```python
from build123d import *

# Parameters (mm, degrees)
SKETCH4_R                = 4.7625
SKETCH4_R_2              = 3.5179
BOSS_EXTRUDE1_DEPTH      = 12.7
BEND_1_OUTLINE_R         = 4.7625
BEND_1_OUTLINE_R_2       = 3.5179
BEND_1_ANGLE             = 90
SKETCH6_R                = 4.7625
SKETCH6_R_2              = 3.5179
POST_BEND_1_LENGTH_DEPTH = 25.4


# Read off the part's stored shape, not the designer's step: Bend 1
with BuildPart() as part:
    # Sketch4 → Boss-Extrude1 (new, symmetric)
    with BuildSketch(Plane(origin=(0, 0, 0), x_dir=(0, 0, -1), z_dir=(1, 0, 0))):
        Circle(SKETCH4_R)
        Circle(SKETCH4_R_2, mode=Mode.SUBTRACT)
    extrude(amount=BOSS_EXTRUDE1_DEPTH, both=True)

    # Bend 1 outline → Bend 1 (revolve)
    with BuildSketch(Plane(origin=(12.7, 0, 11.1125), x_dir=(1, 0, 0), z_dir=(0, 0, 1))):
        with Locations((11.1125, 0)):
            Circle(BEND_1_OUTLINE_R)
        with Locations((11.1125, 0)):
            Circle(BEND_1_OUTLINE_R_2, mode=Mode.SUBTRACT)
    revolve(axis=Axis((12.7, 0, 11.1125), (0, 1, 0)), revolution_arc=BEND_1_ANGLE)

    # Sketch6 → Post Bend 1 Length (add)
    with BuildSketch(Plane.XY.offset(11.1125)):
        with Locations((23.8125, 0)):
            Circle(SKETCH6_R)
        with Locations((23.8125, 0)):
            Circle(SKETCH6_R_2, mode=Mode.SUBTRACT)
    extrude(amount=POST_BEND_1_LENGTH_DEPTH)


solid = part.part
```
Source: CAD feature listing. Evaluate the final solid. Frame: model axes, mm. A direction names the side the tool comes from. Round coordinates to 2 decimals unless told otherwise and drop trailing zeros. Loops run counter-clockwise (first coordinate to the right, second up) from the corner with the lowest first, then second, coordinate; pieces in that order, holes last. Notation, with made-up numbers: (-27.5, 38) - (-11.5, 38) arc R38 cw to (-11.5, 76) - close; hole circle Ø9 at (76.25, 72). An arc over 180 degrees is marked (long way). Use CSV: the item, a comma, the result in double quotes.
Q1. Section query B-B, the plane z = 19.5. Output: boundary loops of the cut face in (x, y) (1 decimal), then the cut area to 3 significant figures.
Reported:
outline,"circle Ø9.5 at (23.8, 0); hole circle Ø7 at (23.8, 0)"
area,"32.4 mm^2"
Q2. Ray query, line 1 along Z through (x, y) = (-6, -0.25); line 2 along Y through (x, z) = (-3, 0); line 3 along X through (y, z) = (-0.25, 25.5). Return the intervals inside material, ascending.
Reported:
line 1,"-4.76 to -3.51, 3.51 to 4.76"
line 2,"-4.76 to -3.52, 3.52 to 4.76"
line 3,"19.06 to 20.3, 27.32 to 28.57"
Q3. Section query C-C, the plane y = 3. Output: boundary loops of the cut face in (x, z).
Reported:
outline,"(-12.7, -3.7) - (12.7, -3.7) arc R14.81 ccw to (27.51, 11.11) - (27.51, 36.51) - (25.65, 36.51) - (25.65, 11.11) arc R12.95 cw to (12.7, -1.84) - (-12.7, -1.84) - close; (-12.7, 1.84) - (12.7, 1.84) arc R9.28 ccw to (21.98, 11.11) - (21.98, 36.51) - (20.11, 36.51) - (20.11, 11.11) arc R7.41 cw to (12.7, 3.7) - (-12.7, 3.7) - close"
Q4. Pin query (flat end, axial travel): pin 1 Ø2 at (y, z) = (3, 13.5) entering from +X; pin 2 Ø4 at (x, y) = (23.81, 0) entering from +Z; pin 3 Ø1 at (x, y) = (1.5, -3.5) entering from -Z. Return the tip coordinate at first contact, or that it passes through.
Reported:
pin 1,"x = 28.13"
pin 2,"z = 4.62"
pin 3,"z = -3.7"
Q5. Section query D-D, the plane x = -7. Output: boundary loops of the cut face in (y, z) (1 decimal).
Reported:
outline,"circle Ø9.5 at (0, 0); hole circle Ø7 at (0, 0)"
Q6. Mould query, pull axis Y, two halves, no side actions, for faces 1 (the flat face through (23, -4, 36.512)), 2 (the cylindrical face through (19.055, 0.209, 23.635)), 3 (the cylindrical face through (27.168, 1.057, 23.635)). Classes: pulls with the +Y half, pulls with the -Y half, needs draft (parallel to the pull), parting line crosses it, or undercut.
Reported:
face 1,"needs draft"
face 2,"parting line crosses it"
face 3,"undercut"
Q7. Reachability of faces 4 (the cylindrical face through (-0.178, 3.488, 0.458)), 5 (the flat face through (-12.7, -4, 0)) from +Z, -Z, +X, -X, +Y, -Y: full face, straight path, thin tool, end or side. Return the list, or none.
Reported:
face 4,"-X"
face 5,"+Z, -Z, -X, +Y, -Y"
